For this review, take the finished solid that the model builds, in its own axes (mm). A direction names the side the tool comes from. Coordinates: 2 decimals unless noted, no trailing zeros. Write each loop counter-clockwise with the first axis right and the second up, starting at its lowest first coordinate (ties: lowest second). Pieces come first, ordered by that corner, then holes. Notation, with made-up numbers: M 17.5,-24.75 L 68.5,-24.75 A24 ccw 68.5,6.25 Z; hole C 34,29.5 d2. An arc over 180 degrees is marked long. Return JSON: item names as keys, results as strings.
```python
from build123d import *

# Parameters (mm, degrees)
SKETCH_R     = 2.2
PAD_DEPTH    = 4
PAD001_DEPTH = 6
POCKET_DEPTH = 2


with BuildPart() as part:
    # Sketch → Pad (new body)
    with BuildSketch(Plane.XY):
        with BuildLine():
            Line((0, 0), (17.4, 0))
            Line((17.4, 0), (17.4, 14.6))
            ThreePointArc((17.4, 14.6), (15.818377, 18.418377), (12, 20))
            Line((12, 20), (0, 20))
            Line((0, 20), (0, 0))
        make_face()
        with Locations((12, 14.6)):
            Circle(SKETCH_R, mode=Mode.SUBTRACT)
    pad = extrude(amount=PAD_DEPTH)

    # Sketch001 → Pad001 (join)
    with BuildSketch(Plane.XZ):
        with BuildLine():
            ThreePointArc((0, 13.8), (3.2, 17), (0, 20.2))
            Line((0, 20.2), (0, 25.973503))
            ThreePointArc((7.861053, 21.327539), (4.565663, 24.725184), (0, 25.973503))
            Line((7.861053, 21.327539), (17.4, 4))
            Line((17.4, 0), (17.4, 4))
            Line((0, 0), (17.4, 0))
            Line((0, 13.8), (0, 0))
        make_face()
    pad001 = extrude(amount=-PAD001_DEPTH)

    # Sketch002 → Pocket (cut)
    with BuildSketch(Plane.XZ.offset(-6)):
        Polygon((0, 22.773503), (-5, 19.886751), (-5, 14.113249), (0, 11.226497), (5, 14.113249), (5, 19.886751), align=None)
    pocket = extrude(amount=POCKET_DEPTH, mode=Mode.SUBTRACT)

    # Mirrored: Pad, Pad001, Pocket across Sketch V_Axis
    add(pad.mirror(Plane(origin=(0, 0, 0), x_dir=(0, 0, 1), z_dir=(1, 0, 0))))
    add(pad001.mirror(Plane(origin=(0, 0, 0), x_dir=(0, 0, 1), z_dir=(1, 0, 0))))
    add(pocket.mirror(Plane(origin=(0, 0, 0), x_dir=(0, 0, 1), z_dir=(1, 0, 0))), mode=Mode.SUBTRACT)


solid = part.part
```
1. We need section A-A (z = 16.25). State the section outline as (x, y) points.
Checks:
{"outline": "M -10.66,0 L -3.11,0 L -3.11,4 L -5,4 L -5,6 L -10.66,6 Z; M 3.11,0 L 10.66,0 L 10.66,6 L 5,6 L 5,4 L 3.11,4 Z"}
2. Draft analysis for pull direction X (two halves, no side actions). For faces 4 (the face through (15.86, 18.376, 1.972)), 5 (the face through (-12.56, 2.96, 12.79)), 6 (the face through (-2.465, 5.014, 12.65)), state which applies: +X half, -X half, draft (parallel to the pull), parting line (faces both ways), or undercut.
Checks:
{"face 4": "+X half", "face 5": "-X half", "face 6": "undercut"}
3. For faces 1 (the face through (-15.86, 18.376, 1.972)), 2 (the face through (0, 13, 4)), 3 (the face through (5, 5, 17)), list the 3-axis set-ups (+Z, -Z, +X, -X, +Y, -Y) from which the entire face can be reached by the end or side of a thin tool; tool diameter is ignored.
Checks:
{"face 1": "+Z, -Z, -X, +Y", "face 2": "+Z, +X, -X, +Y", "face 3": "+Y"}
4. We need section D-D (z = 11.75). State the section outline as (x, y) points, plus the area to 3 significant figures.
Checks:
{"outline": "M -13.13,0 L 13.13,0 L 13.13,6 L 0.91,6 L 0.91,4 L -0.91,4 L -0.91,6 L -13.13,6 Z", "area": "154 mm2"}
5. Wall thickness on L1, parallel to Y at x = -12, z = 3.05; L2, parallel to X at y = 15.25, z = 2; L3, parallel to Z at x = -2, y = 11.25: over which ranges is each line inside the solid? List them lowest first. Write a range as from..to.
Checks:
{"L1": "0..12.4, 16.8..20", "L2": "-17.36..-14.1, -9.9..9.9, 14.1..17.36", "L3": "0..4"}
6. Clearance check with flat-ended pins moving along their axes: pin 1 Ø4 at (x, z) = (-12, 12.5) entering from -Y; pin 2 Ø5 at (x, z) = (1, 17) entering from +Y; pin 3 Ø2 at (x, z) = (9, 20.5) entering from +Y; pin 4 Ø6 at (x, y) = (6, 3.5) entering from +Z. State where each tip first meets the part, or that it passes through.
Checks:
{"pin 1": "y = 0", "pin 2": "y = 4", "pin 3": "y = 6", "pin 4": "z = 25.46"}
7. We need section B-B (y = 1.5). State the section outline as (x, z) points.
Checks:
{"outline": "M -17.4,0 L 17.4,0 L 17.4,4 L 7.86,21.33 A8.97 ccw 0,25.97 A8.97 ccw -7.86,21.33 L -17.4,4 Z; hole C 0,17 d6.4"}
8. We need section C-C (y = 13.5). State the section outline as (x, z) points.
Checks:
{"outline": "M -17.4,0 L -13.91,0 L -13.91,4 L -17.4,4 Z; M -10.09,0 L 10.09,0 L 10.09,4 L -10.09,4 Z; M 13.91,0 L 17.4,0 L 17.4,4 L 13.91,4 Z"}
